Input: part model. Units: mm. Frame: model coordinates. Give positions to 0.01 mm unless a question says otherwise; leave off trailing zeros. Order: outer loops, then holes, each group sorted by start corner. A loop starts at its lowest first (then second) coordinate and runs counter-clockwise, first axis right, second up. Notation, with made-up numbers: M 27,-8.5 L 86,-8.5 A18 cw 86,9.5 Z; hole C 41.25,45 d11. An arc over 180 degrees is marked long. Use a Markdown table: item, result.
from build123d import *

# Parameters (mm, degrees)
F1_DEPTH = 6
F2_R     = 5
F3_R     = 0.2
F4_R     = 0.2


with BuildPart() as f1:
    # F0 (on Top) → F1 (new body)
    with BuildSketch(Plane.XY):
        with BuildLine():
            Line((10.75, -18.6195461814), (0, 0))
            Line((0, 0), (-10.75, -18.6195461814))
            ThreePointArc((-10.75, -18.6195461814), (0, -21.5), (10.75, -18.6195461814))
        make_face()
    extrude(amount=F1_DEPTH)

    # F2
    f2_edges = [f1.edges().sort_by_distance(p)[0] for p in [
        (0, 0, 3),
    ]]
    fillet(f2_edges, radius=F2_R)

    # F3
    f3_edges = [f1.edges().sort_by_distance(p)[0] for p in [
        (7.540064, -13.059773, 6),
        (0, -5, 6),
        (0, -21.5, 6),
        (-7.540064, -13.059773, 6),
    ]]
    fillet(f3_edges, radius=F3_R)

    # F4
    f4_edges = [f1.edges().sort_by_distance(p)[0] for p in [
        (7.540064, -13.059773, 0),
        (0, -5, 0),
        (0, -21.5, 0),
        (-7.540064, -13.059773, 0),
    ]]
    fillet(f4_edges, radius=F4_R)


solid = f1.part
1) Cut plane A-A on z = 0.75. Return loops of the section in (x, y), and give its area (3 significant figures).
Response values:
| item | result |
|---|---|
| outline | M -10.75,-18.62 A21.5 ccw 10.75,-18.62 L 4.33,-7.5 A5 ccw -4.33,-7.5 Z |
| area | 225 mm² |
2) Material intervals for line 1 (X direction, y = -7.5, z = 0.5); line 2 (X direction, y = -14, z = 4); line 3 (Y direction, x = 1, z = 5.25), sorted ascending. Write a range as from..to.
Response values:
| item | result |
|---|---|
| line 1 | x = -4.33..4.33 |
| line 2 | x = -8.08..8.08 |
| line 3 | y = -21.48..-5.1 |
3) First-contact query: pin 1 Ø2 at (x, z) = (-1.5, 4) entering from +Y; pin 2 Ø2 at (x, z) = (8.5, 2) entering from -Y; pin 3 Ø1 at (x, z) = (-1.5, 3.5) entering from +Y; pin 4 Ø1.5 at (y, z) = (-19, 2) entering from +X. Flat tips, straight axial feed; report the tip coordinate or a pass-through.
Response values:
| item | result |
|---|---|
| pin 1 | stops at y = -5.03 |
| pin 2 | stops at y = -20.15 |
| pin 3 | stops at y = -5.1 |
| pin 4 | stops at x = 10.75 |
